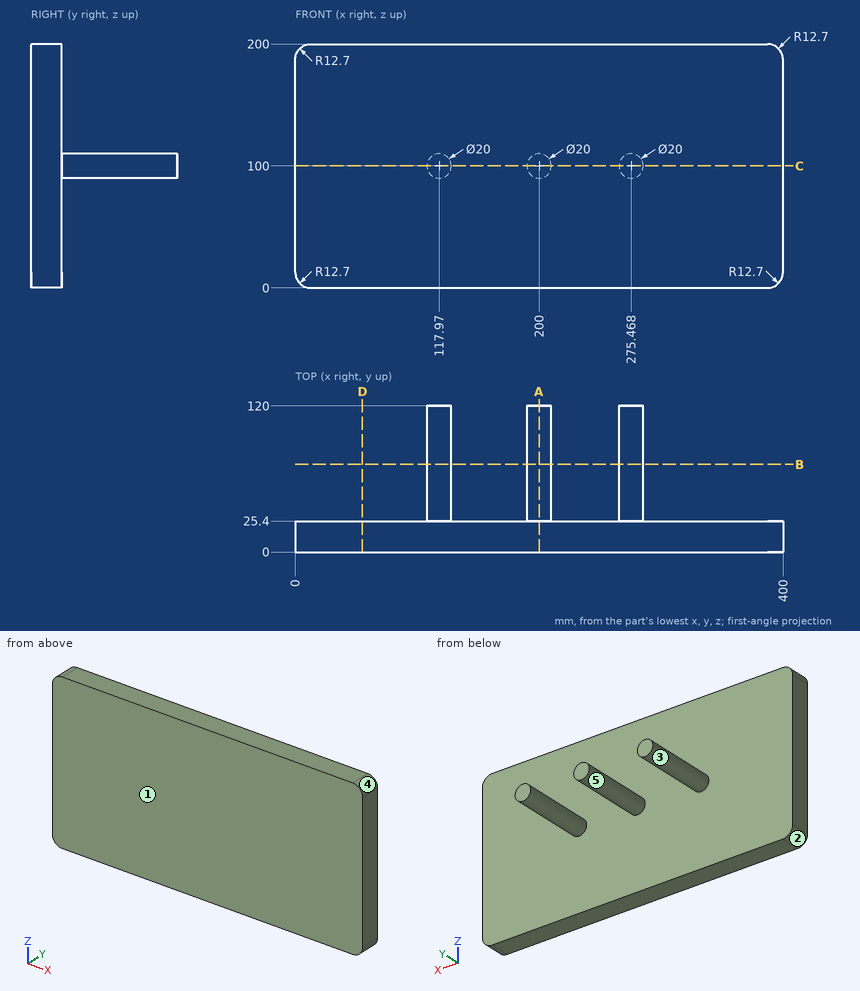
Job drawing, mm, ordinate dimensions from the low corner. One solid piece. A direction names the side the tool comes from. Give positions to 0.01 mm unless a question says otherwise; leave off trailing zeros. Loops run counter-clockwise (first coordinate to the right, second up) from the corner with the lowest first, then second, coordinate; pieces in that order, holes last. Notation, with made-up numbers: (59, -33) -> (97, -33) arc R27 ccw to (97, 0) -> close; hole circle Ø10 at (1, -24). An arc over 180 degrees is marked (long way). Write each question's results on one line, items separated by ' | '. Start each with the question number.
Q1. Pin check, flat tip, straight feed: P1, Ø1, axis at x = 158, z = 123.5, coming from the +Y side. Stop position of the tip, or through.
Q2. Pull direction X, two halves, no side cores. Call the marked faces 1, 2 and 3: +X half, -X half, draft (parallel to the pull), parting line (faces both ways), or undercut.
Q3. Band-saw the part on C-C on z = 100. List the corners of the cut face in (x, y), plus the area to 3 significant figures.
Q4. Band-saw the part on D-D on x = 55. List the corners of the cut face in (y, z).
Q5. Band-saw the part on A-A on x = 200. List the corners of the cut face in (y, z).
Q6. Wall check: L1, parallel to Y at x = 202, z = 64. Give the ranges that are in metal, low to high.
Q7. Which spindle directions (+Z, -Z, +X, -X, +Y, -Y) get a long thin tool onto all of the face, cutting with end or side? Do the marked faces 4 and 5. Say none if no direction does.
Q8. Band-saw the part on B-B on y = 72. List the corners of the cut face in (x, z).
Results are:
1) P1: stops at y = 25.4
2) face 1: draft | face 2: -X half | face 3: undercut
3) outline: (0, 0) -> (400, 0) -> (400, 25.4) -> (285.47, 25.4) -> (285.47, 120) -> (265.47, 120) -> (265.47, 25.4) -> (210, 25.4) -> (210, 120) -> (190, 120) -> (190, 25.4) -> (127.97, 25.4) -> (127.97, 120) -> (107.97, 120) -> (107.97, 25.4) -> (0, 25.4) -> close | area: 15,800 mm²
4) outline: (0, 0) -> (25.4, 0) -> (25.4, 200) -> (0, 200) -> close
5) outline: (0, 0) -> (25.4, 0) -> (25.4, 90) -> (120, 90) -> (120, 110) -> (25.4, 110) -> (25.4, 200) -> (0, 200) -> close
6) L1: y = 0 to 25.4
7) face 4: +Z, +X, +Y, -Y | face 5: +Y
8) outline: circle Ø20 at (117.97, 100); circle Ø20 at (200, 100); circle Ø20 at (275.47, 100)
